Check sheet for the modelled part. Datum: model origin and axes. Units: mm. A direction names the side the tool comes from. Coordinates: 2 decimals unless noted, no trailing zeros. Write each loop counter-clockwise with the first axis right and the second up, starting at its lowest first coordinate (ties: lowest second). Pieces come first, ordered by that corner, then holes. Notation, with made-up numbers: (39.5, 40.25) -> (91.5, 40.25) arc R11 cw to (91.5, 60.25) -> close; hole circle Ø3 at (57.25, 88.5). An arc over 180 degrees is marked (long way). One line per item, written item: value. Start each with the question number.
1) Draft check along X on faces 1 (the flat face through (60.514, 15.465, -3.451)), 2 (the flat face through (54.239, 9, -22)), 3 (the flat face through (25, -13, -29)). Enter one of: +X half, -X half, draft (parallel to the pull), parting line (faces both ways), or undercut.
2) Set-up check for faces 4 (the flat face through (20, -11.25, -18)), 5 (the flat face through (0, -14, -22)), 6 (the flat face through (21, -1, 0)): record each of +Z, -Z, +X, -X, +Y, -Y from which the full face is reachable in a straight line by a thin tool's end or side.
3) Sectioned sample at D-D on z = -10.5. Enter the section's corners in (x, y).
4) Scan lines: line 1 along X through (y, z) = (12, -25); line 2 along Y through (x, z) = (56, -25.5); line 3 along Y through (x, z) = (11.35, -6.5). Record each from-to range of solid material in increasing order. Write a range as [from, to].
5) Sectioned sample at C-C on y = 9. Enter the section's corners in (x, z), plus the area to 3 significant figures.
6) Gauge pin test, flat ends, axial feed: P1, Ø1, axis at x = 52.5, z = -22.5, coming from the +Y side; P2, Ø4, axis at x = 48.5, y = 13.5, coming from the -Z side; P3, Ø8, axis at x = 42, z = -11.5, coming from the +Y side. Record the tip position at first contact, or that the pin passes through.
7) Sectioned sample at B-B on x = 0. Enter the section's corners in (y, z).
8) Sectioned sample at A-A on y = 0. Enter the section's corners in (x, z), plus the area to 3 significant figures.
```python
from build123d import *

# Parameters (mm, degrees)
SKETCH1_R           = 5.35
BOSS_EXTRUDE2_DEPTH = 7
SKETCH8_R           = 2
CUT_EXTRUDE2_DEPTH  = 2.25
BOSS_EXTRUDE3_DEPTH = 22
SKETCH10_W          = 82.482524805
SKETCH10_H          = 7
BOSS_EXTRUDE4_DEPTH = 5
CHAMFER1_SIZE       = 5
SKETCH11_W          = 28.790613911
SKETCH11_H          = 3
SKETCH11_W_2        = 32.450648491
CUT_EXTRUDE3_DEPTH  = 15


with BuildPart() as part:
    # Sketch1 → Boss-Extrude2 (new body)
    with BuildSketch(Plane.XY):
        Polygon((-19.503784034, -20), (19.503784034, -20), (62.978740771, -20), (62.978740771, 13), (19.503784034, 13), (-19.503784034, 13), align=None)
        Circle(SKETCH1_R, mode=Mode.SUBTRACT)
    extrude(amount=-BOSS_EXTRUDE2_DEPTH)

    # Sketch8 → Cut-Extrude2 (cut)
    with BuildSketch(Plane(origin=(0, 0, -7), x_dir=(-1, 0, 0), z_dir=(0, 0, -1))):
        with Locations((-11.35, 0)):
            Circle(SKETCH8_R)
    extrude(amount=-CUT_EXTRUDE2_DEPTH, mode=Mode.SUBTRACT)

    # Sketch9 → Boss-Extrude3 (add)
    with BuildSketch(Plane(origin=(0, 0, -7), x_dir=(-1, 0, 0), z_dir=(0, 0, -1))):
        Polygon((11.5, 3.25), (11.5, 13), (19.503784034, 13), (19.503784034, -12.662545792), (19.503784034, -20), (-56.5, -20), (-62.978740771, -20), (-62.978740771, 13), (-51.5, 13), (-51.5, 5), (-53.5, 5), (-53.5, -5), (-51.5, -5), (-51.5, -11.25), (11.5, -11.25), (11.5, -3.25), (16.5, -3.25), (16.5, 3.25), align=None)
    extrude(amount=BOSS_EXTRUDE3_DEPTH)

    # Sketch10 → Boss-Extrude4 (add)
    with BuildSketch(Plane(origin=(0, 13, 0), x_dir=(1, 0, 0), z_dir=(0, 1, 0))):
        with Locations((21.737478368, 3.5)):
            Rectangle(SKETCH10_W, SKETCH10_H)
    extrude(amount=BOSS_EXTRUDE4_DEPTH)

    # Chamfer1
    chamfer1_edges = [part.edges().sort_by_distance(p)[0] for p in [
        (62.978740771, 18, -3.5),
        (-19.503784034, 18, -3.5),
    ]]
    chamfer(chamfer1_edges, length=CHAMFER1_SIZE)

    # Sketch11 → Cut-Extrude3 (cut)
    with BuildSketch(Plane(origin=(0, 0, -29), x_dir=(-1, 0, 0), z_dir=(0, 0, -1))):
        Polygon((-60.239370385, 10), (-58.239370385, 10), (-58.239370385, 13), (-56.239370385, 13), (-56.239370385, 10), (-54.239370385, 10), (-54.239370385, 8), (-60.239370385, 8), align=None)
        with Locations((-45.84406343, -15.5)):
            Rectangle(SKETCH11_W, SKETCH11_H)
        with Locations((0.276567771, -15.5)):
            Rectangle(SKETCH11_W_2, SKETCH11_H)
        Polygon((14.501892017, 13), (16.501892017, 13), (16.501892017, 10), (18.501892017, 10), (18.501892017, 8), (12.501892017, 8), (12.501892017, 10), (14.501892017, 10), align=None)
    extrude(amount=-CUT_EXTRUDE3_DEPTH, mode=Mode.SUBTRACT)


solid = part.part
```
Answers:
1. face 1: +X half
1. face 2: undercut
1. face 3: draft
2. face 4: -Z, +Y
2. face 5: -Z
2. face 6: +Z, +X, -X, +Y, -Y
3. outline: (-19.5, -20) -> (62.98, -20) -> (62.98, 13) -> (51.5, 13) -> (51.5, 5) -> (53.5, 5) -> (53.5, -5) -> (51.5, -5) -> (51.5, -11.25) -> (-11.5, -11.25) -> (-11.5, -3.25) -> (-16.5, -3.25) -> (-16.5, 3.25) -> (-11.5, 3.25) -> (-11.5, 13) -> (-19.5, 13) -> close
4. line 1: x = [-19.5, -16.5], [-14.5, -11.5], [51.5, 56.24], [58.24, 62.98]
4. line 2: y = [-20, -17], [-14, 8], [10, 13]
4. line 3: y = [-20, -2], [2, 18]
5. outline: (-19.5, -29) -> (-18.5, -29) -> (-18.5, -14) -> (-12.5, -14) -> (-12.5, -29) -> (-11.5, -29) -> (-11.5, -7) -> (51.5, -7) -> (51.5, -29) -> (54.24, -29) -> (54.24, -14) -> (60.24, -14) -> (60.24, -29) -> (62.98, -29) -> (62.98, 0) -> (-19.5, 0) -> close
5. area: 826 mm2
6. P1: stops at y = 13
6. P2: stops at z = -7
6. P3: stops at y = -11.25
7. outline: (-20, -29) -> (-17, -29) -> (-17, -14) -> (-14, -14) -> (-14, -29) -> (-11.25, -29) -> (-11.25, -7) -> (-5.35, -7) -> (-5.35, 0) -> (-20, 0) -> close; (5.35, -7) -> (18, -7) -> (18, 0) -> (5.35, 0) -> close
8. outline: (-19.5, -29) -> (-16.5, -29) -> (-16.5, -7) -> (-5.35, -7) -> (-5.35, 0) -> (-19.5, 0) -> close; (5.35, -7) -> (9.35, -7) -> (9.35, -4.75) -> (13.35, -4.75) -> (13.35, -7) -> (53.5, -7) -> (53.5, -29) -> (62.98, -29) -> (62.98, 0) -> (5.35, 0) -> close
8. area: 768 mm2
